Autodesk Inventor part; units mm, degrees
ref_plane "YZ Plane" through (0, 0, 0) normal (1, 0, 0) x (0, 1, 0)
ref_plane "XZ Plane" through (0, 0, 0) normal (0, 1, 0) x (-1, 0, 0)
ref_plane "XY Plane" through (0, 0, 0) normal (0, 0, 1) x (1, 0, 0)
sketch "Sketch1" plane through (0, 0, 0) normal (0, 0, 1) x (1, 0, 0)
  circle A0 centre (0, 0) radius 6.5
  dimension "d0" = 13
extrude "Extrusion1" add sketch "Sketch1" along normal blind 10
sketch "Sketch2" plane through (0, 0, 10) normal (0, 0, 1) x (1, 0, 0)
  circle A0 centre (0, 0) radius 5
  dimension "d3" = 10
extrude "Extrusion2" cut sketch "Sketch2" against normal blind 8
sketch "Sketch3" plane through (0, 0, 10) normal (0, 0, 1) x (1, 0, 0)
  circle A0 centre (0, 0) radius 5
  circle A1 centre (0, 0) radius 6.5
  line L0 (-2, 0) -> (2, 0)
  line L1 (2, 0) -> (2, -6.9117)
  line L2 (2, -6.9117) -> (-2, -6.9117)
  line L3 (-2, -6.9117) -> (-2, 0)
  dimension "d6" = 4
extrude "Extrusion3" cut sketch "Sketch3" against normal blind 4 contours L3 L0 L1 A0 | A0 L1 A1 L3 | A1 L1 L2 L3 picked at (0, -1.6667) picked at (-1.2327, -5.848)
properties part number "capuchon.torre0.2"
Here's how the part is built. I have some questions about the finished solid (model axes, mm). A direction names the side the tool comes from. Round coordinates to 2 decimals unless told otherwise and drop trailing zeros. Write each loop counter-clockwise with the first axis right and the second up, starting at its lowest first coordinate (ties: lowest second). Pieces come first, ordered by that corner, then holes.
Q1. If we mould it in two halves opening along Y, with no side actions, what happens to faces 4 (the cylindrical face through (-1.409, 6.345, 4.93)), 5 (the flat face through (0, -6, 6)), 6 (the cylindrical face through (3, 4, 6))? For each: +Y half, -Y half, draft (parallel to the pull), parting line (faces both ways), or undercut.
Q2. If we section it at C-C on z = 4: Write out the boundary of the cut face in (x, y).
Q3. Please list where these lines run through material, in increasing order: probe 1 along Y at (x, z) = (0, 5.5); probe 2 along Y at (x, z) = (0, 7).
Q4. If we section it at B-B on y = 0: Write out the boundary of the cut face in (x, z), plus the area to 3 significant figures.
Q5. If we section it at A-A on x = 0: Write out the boundary of the cut face in (y, z), plus the area to 3 significant figures.
Q6. Will these pins go through, and if not, where does the flat tip stop? P1, Ø4, axis at x = 2.5, z = 6.5, coming from the -Y side; P2, Ø2, axis at x = -2.5, z = 3.5, coming from the +Y side; P3, Ø1.8, axis at y = -5, z = 8, coming from the +X side.
Q7. Which directions (+Z, -Z, +X, -X, +Y, -Y) give clear straight access to the entire face, cutting with the end or side of a thin tool? Please do faces 1 (the flat face through (0, 0, 2)), 2 (the flat face through (-2, -5, 8)), 3 (the flat face through (-2, 5, 10)).
Answer below:
1. face 4: parting line
1. face 5: draft
1. face 6: undercut
2. outline: circle Ø13 at (0, 0); hole circle Ø10 at (0, 0)
3. probe 1: y = -6.5 to -5, 5 to 6.5
3. probe 2: y = 5 to 6.5
4. outline: (-6.5, 0) - (6.5, 0) - (6.5, 10) - (5, 10) - (5, 2) - (-5, 2) - (-5, 10) - (-6.5, 10) - close
4. area: 50.0 mm2
5. outline: (-6.5, 0) - (6.5, 0) - (6.5, 10) - (5, 10) - (5, 2) - (-5, 2) - (-5, 6) - (-6.5, 6) - close
5. area: 44.0 mm2
6. P1: stops at y = -6.48
6. P2: stops at y = 6.32
6. P3: stops at x = 5.04
7. face 1: +Z
7. face 2: +Z, -Y
7. face 3: +Z, +X, -X, +Y, -Y
